```python
from build123d import *

# Parameters (mm, degrees)
M8_TAPPED_HOLE1_D           = 6.8
M8_TAPPED_HOLE1_DEPTH       = 16.75
M8_TAPPED_HOLE1_CSINK_D     = 8.05
M8_TAPPED_HOLE1_CSINK_ANGLE = 90
M8_TAPPED_HOLE1_TIP         = 2.042926105


with BuildPart() as part:
    # Sketch1 → Revolve1 (revolve)
    with BuildSketch(Plane.XY, mode=Mode.PRIVATE) as revolve1_sk:
        with BuildLine():
            Line((0, 0), (47.5, 0))
            Line((47.5, 0), (47.5, 8))
            Line((47.5, 8), (43.5, 8))
            Line((43.5, 8), (43.5, 15))
            Line((43.5, 15), (47.5, 15))
            Line((47.5, 15), (47.5, 305.5))
            ThreePointArc((47.5, 305.5), (45, 308), (47.5, 310.5))
            Line((47.5, 310.5), (47.5, 332))
            Line((47.5, 332), (25, 332))
            Line((25, 332), (25, 82))
            Line((25, 82), (0, 82))
            Line((0, 82), (0, 0))
        make_face()
    revolve(revolve1_sk.sketch.rotate(Axis((0, 0, 0), (0, 1, 0)), 90), axis=Axis((0, 0, 0), (0, 1, 0)))

    # M8 Tapped Hole1
    with Locations(Plane(origin=(21.213203436, 0, 21.213203436), x_dir=(0, 0, -1), z_dir=(0, -1, 0))):
        with Locations((0, 0), (0, -42.426406872), (42.426406872, -42.426406872), (42.426406872, 0)):
            CounterSinkHole(M8_TAPPED_HOLE1_D / 2, M8_TAPPED_HOLE1_CSINK_D / 2, depth=M8_TAPPED_HOLE1_DEPTH, counter_sink_angle=M8_TAPPED_HOLE1_CSINK_ANGLE)
            with Locations((0, 0, -(M8_TAPPED_HOLE1_DEPTH + M8_TAPPED_HOLE1_TIP / 2))):  # 118° drill point
                Cone(0, M8_TAPPED_HOLE1_D / 2, M8_TAPPED_HOLE1_TIP, mode=Mode.SUBTRACT)


solid = part.part
```
Geometry check sheet. Reference: the model listing, model coordinates, mm. A direction names the side the tool comes from. Round coordinates to 2 decimals unless told otherwise and drop trailing zeros. Loops run counter-clockwise (first coordinate to the right, second up) from the corner with the lowest first, then second, coordinate; pieces in that order, holes last. Notation, with made-up numbers: M 86,88 L 118,88 A7 ccw 118,94 Z; hole C 47.5,16.25 d9. An arc over 180 degrees is marked long. Return JSON: item names as keys, results as strings. Group by question number.
(1) Mould release check, pull along Y, two halves, no side actions. Record for faces 1 (the face through (38.5, 8, -20.9)), 2 (the face through (-20.814, 18.438, 21.648)), 3 (the face through (46.37, 321.4, 10.3)): pulls with the +Y half, pulls with the -Y half, needs draft (parallel to the pull), parting line crosses it, or undercut.
(2) Scan lines: line 1 along Z through (x, y) = (-0.5, 154.5) (3 decimals); line 2 along Y through (x, z) = (1, 12); line 3 along X through (y, z) = (217, 0). Record each from-to range of solid material in increasing order. Write a range as [from, to].
(3) Set-up check for faces 4 (the face through (-43.13, 11.55, 5.66)), 5 (the face through (-7.509, 205.25, -23.846)), 6 (the face through (23.511, 8.8, 18.707)): record each of +Z, -Z, +X, -X, +Y, -Y from which the full face is reachable in a straight line by a thin tool's end or side.
(4) Section check B-B, the plane x = 0. Enter the section's corners in (y, z).
(5) Section check A-A, the plane z = 0. Enter the section's corners in (x, y), and give its area (3 significant figures).
(6) Section check D-D, the plane y = 75. Enter the section's corners in (x, z), and give its area (3 significant figures).
(7) Go/stop test with flat-tipped pins: pin 1 (5 mm diameter, centred on x = 10, y = 125.5, fed in from +Z); pin 2 (8 mm diameter, centred on x = 28.5, y = 286.5, fed in from +Z); pin 3 (8 mm diameter, centred on y = 62, z = 1, fed in from +X). Record where each tip stops, or that it passes through.
(8) Section check C-C, the plane y = 164. Enter the section's corners in (x, z), and give its area (3 significant figures).
Data:
{
 "1": {"face 1": "undercut", "face 2": "pulls with the -Y half", "face 3": "needs draft"},
 "2": {"line 1": "[-47.497, -24.995], [24.995, 47.497]", "line 2": "[0, 82]", "line 3": "[-47.5, -25], [25, 47.5]"},
 "3": {"face 4": "none", "face 5": "+Y", "face 6": "-Y"},
 "4": {"outline": "M 0,-47.5 L 8,-47.5 L 8,-43.5 L 15,-43.5 L 15,-47.5 L 305.5,-47.5 A2.5 cw 310.5,-47.5 L 332,-47.5 L 332,-25 L 82,-25 L 82,25 L 332,25 L 332,47.5 L 310.5,47.5 A2.5 cw 305.5,47.5 L 15,47.5 L 15,43.5 L 8,43.5 L 8,47.5 L 0,47.5 Z"},
 "5": {"outline": "M -47.5,0 L 47.5,0 L 47.5,8 L 43.5,8 L 43.5,15 L 47.5,15 L 47.5,305.5 A2.5 cw 47.5,310.5 L 47.5,332 L 25,332 L 25,82 L -25,82 L -25,332 L -47.5,332 L -47.5,310.5 A2.5 cw -47.5,305.5 L -47.5,15 L -43.5,15 L -43.5,8 L -47.5,8 Z", "area": "19,000 mm²"},
 "6": {"outline": "C 0,0 d95", "area": "7,090 mm²"},
 "7": {"pin 1": "z = 46.9", "pin 2": "z = 40.69", "pin 3": "x = 47.5"},
 "8": {"outline": "C 0,0 d95; hole C 0,0 d50", "area": "5,120 mm²"}
}
